Geometry check sheet. Reference: the model listing, model coordinates, mm. A direction names the side the tool comes from. Coordinates: 2 decimals unless noted, no trailing zeros. Write each loop counter-clockwise with the first axis right and the second up, starting at its lowest first coordinate (ties: lowest second). Pieces come first, ordered by that corner, then holes. Notation, with made-up numbers: (83.5, -37.5) - (105.5, -37.5) arc R22 cw to (105.5, -13.5) - close; hole circle Ø4 at (28.25, -32). An arc over 180 degrees is marked (long way). Answer as a JSON object with one key per item and string values. Group by question number.
from build123d import *

# Parameters (mm, degrees)
F1_DEPTH  = 76.2
F2_DEPTH  = 12.7
F3_W      = 31.496
F3_H      = 7.874
F4_DEPTH  = 38.101
F6_DEPTH  = 63.501
F7_W      = 31.496
F7_H      = 25.4
F8_DEPTH  = 55.627
F9_W      = 28.702
F9_H      = 25.4
F10_DEPTH = 63.501
F11_R     = 7.112
F12_DEPTH = 38.101
F11_R_2   = 12.7
F13_DEPTH = 4.572


with BuildPart() as f1:
    # F0 (on Right) → F1 (new body)
    with BuildSketch(Plane.YZ):
        Polygon((-31.75, 38.1), (-31.75, 0), (-19.05, 0), (-19.05, 6.35), (19.05, 6.35), (19.05, 0), (31.75, 0), (31.75, 38.1), align=None)
    extrude(amount=F1_DEPTH)

    # F0 (on Right) → F2 (join)
    with BuildSketch(Plane.YZ):
        with BuildLine():
            Line((-31.75, 47.752), (-31.75, 38.1))
            Line((-31.75, 38.1), (31.75, 38.1))
            Line((31.75, 38.1), (31.75, 47.752))
            ThreePointArc((31.75, 47.752), (28.0302561211, 56.7322561211), (19.05, 60.452))
            Line((19.05, 60.452), (-19.05, 60.452))
            ThreePointArc((-19.05, 60.452), (-28.0302561211, 56.7322561211), (-31.75, 47.752))
        make_face()
        with BuildLine():
            ThreePointArc((-19.05, 48.5814124708), (-22.987, 52.5184124708), (-19.05, 56.4554124708))
            Line((-19.05, 56.4554124708), (19.05, 56.4554124708))
            ThreePointArc((19.05, 56.4554124708), (21.8338793975, 55.3022918683), (22.987, 52.5184124708))
            ThreePointArc((22.987, 52.5184124708), (21.8338793975, 49.7345330733), (19.05, 48.5814124708))
            Line((19.05, 48.5814124708), (-19.05, 48.5814124708))
        make_face(mode=Mode.SUBTRACT)
    extrude(amount=F2_DEPTH)

    # F3 (on face) → F4 (cut, through all)
    with BuildSketch(Plane.XY.offset(38.1)):
        with Locations((44.45, 27.813)):
            Rectangle(F3_W, F3_H)
        with Locations((44.45, -27.813)):
            Rectangle(F3_W, F3_H)
    extrude(amount=-F4_DEPTH, mode=Mode.SUBTRACT)

    # F5 (on face) → F6 (cut, through all)
    with BuildSketch(Plane.XZ.offset(31.75)):
        Polygon((60.198, 0), (63.5, 0), (63.5, 25.4), (62.9462525249, 25.4), (60.198, 25.4), align=None)
    extrude(amount=-F6_DEPTH, mode=Mode.SUBTRACT)

    # F7 (on face) → F8 (cut, through all)
    with BuildSketch(Plane.XZ.offset(23.876)):
        with Locations((44.45, 12.7)):
            Rectangle(F7_W, F7_H)
    extrude(amount=-F8_DEPTH, mode=Mode.SUBTRACT)

    # F9 (on face) → F10 (cut, through all)
    with BuildSketch(Plane.XZ.offset(31.75)):
        with Locations((14.351, 12.7)):
            Rectangle(F9_W, F9_H)
    extrude(amount=-F10_DEPTH, mode=Mode.SUBTRACT)

    # F11 (on face) → F12 (cut, through all)
    with BuildSketch(Plane.XY.offset(38.1)):
        with Locations((44.45, 0)):
            Circle(F11_R)
    extrude(amount=-F12_DEPTH, mode=Mode.SUBTRACT)

    # F11 (on face) → F13 (cut)
    with BuildSketch(Plane.XY.offset(38.1)):
        with Locations((44.45, 0)):
            Circle(F11_R_2)
        with Locations((44.45, 0)):
            Circle(F11_R, mode=Mode.SUBTRACT)
    extrude(amount=-F13_DEPTH, mode=Mode.SUBTRACT)


solid = f1.part
(1) Section check B-B (y = 0). Record the cut outline in (x, z).
(2) Draft check along X on faces 1 (the face through (28.702, -28, 32)), 2 (the face through (70, 25, 0)), 3 (the face through (12.7, 0, 47)). Enter one of: +X half, -X half, draft (parallel to the pull), parting line (faces both ways), or undercut.
(3) Section check A-A (x = 44.45). Record the cut outline in (y, z).
(4) Set-up check for faces 4 (the face through (44, -14, 38.1)), 5 (the face through (28.702, 28, 32)), 6 (the face through (6, 0, 48.581)), 7 (the face through (44, -23.876, 32)): record each of +Z, -Z, +X, -X, +Y, -Y from which the full face is reachable in a straight line by a thin tool's end or side.
(5) Section check D-D (y = -22). Record the cut outline in (x, z), and give its area (3 significant figures).
(6) Gauge pin test, flat ends, axial feed: pin 1 (4 mm diameter, centred on x = 33, y = 12, fed in from +Z); pin 2 (10 mm diameter, centred on x = 48, z = 29, fed in from -Y); pin 3 (14 mm diameter, centred on x = 70.5, y = 4, fed in from -Z); pin 4 (18 mm diameter, centred on y = 6, z = 44, fed in from +X). Record the tip position at first contact, or that the pin passes through.
(7) Material ranges on L1, parallel to Y at x = 44.45, z = 28.5; L2, parallel to X at y = 25.5, z = 29; L3, parallel to Y at x = 44, z = 35, recorded low to high. Write a range as [from, to].
(8) Section check C-C (z = 28.5). Record the cut outline in (x, y), and give its area (3 significant figures).
Conclusion:
{
 "1": {"outline": "(0, 25.4) - (37.34, 25.4) - (37.34, 33.53) - (31.75, 33.53) - (31.75, 38.1) - (12.7, 38.1) - (12.7, 48.58) - (0, 48.58) - close; (0, 56.46) - (12.7, 56.46) - (12.7, 60.45) - (0, 60.45) - close; (51.56, 25.4) - (63.5, 25.4) - (63.5, 6.35) - (76.2, 6.35) - (76.2, 38.1) - (57.15, 38.1) - (57.15, 33.53) - (51.56, 33.53) - close"},
 "2": {"face 1": "undercut", "face 2": "draft", "face 3": "+X half"},
 "3": {"outline": "(-23.88, 25.4) - (-7.11, 25.4) - (-7.11, 33.53) - (-12.7, 33.53) - (-12.7, 38.1) - (-23.88, 38.1) - close; (7.11, 25.4) - (23.88, 25.4) - (23.88, 38.1) - (12.7, 38.1) - (12.7, 33.53) - (7.11, 33.53) - close"},
 "4": {"face 4": "+Z, +X, +Y, -Y", "face 5": "+Z, -Z, +Y", "face 6": "+X, -X", "face 7": "+Z, -Z, -Y"},
 "5": {"outline": "(0, 25.4) - (63.5, 25.4) - (63.5, 0) - (76.2, 0) - (76.2, 38.1) - (12.7, 38.1) - (12.7, 49.91) - (0, 49.91) - close; (0, 55.13) - (12.7, 55.13) - (12.7, 60.1) - (0, 60.1) - close", "area": "1,500 mm^2"},
 "6": {"pin 1": "stops at z = 38.1", "pin 2": "stops at y = -23.88", "pin 3": "stops at z = 6.35", "pin 4": "stops at x = 76.2"},
 "7": {"L1": "y = [-23.88, -7.11], [7.11, 23.88]", "L2": "x = [0, 28.7], [60.2, 76.2]", "L3": "y = [-23.88, -12.69], [12.69, 23.88]"},
 "8": {"outline": "(0, -31.75) - (28.7, -31.75) - (28.7, -23.88) - (60.2, -23.88) - (60.2, -31.75) - (76.2, -31.75) - (76.2, 31.75) - (60.2, 31.75) - (60.2, 23.88) - (28.7, 23.88) - (28.7, 31.75) - (0, 31.75) - close; hole circle Ø14.22 at (44.45, 0)", "area": "4,180 mm^2"}
}
